from build123d import *

# Parameters (mm, degrees)
CROQUIS2_R              = 9.365
CROQUIS2_R_2            = 4.87
SALIENTE_EXTRUIR1_DEPTH = 0.2
CORTAR_EXTRUIR1_DEPTH   = 0.1


with BuildPart() as part:
    # Croquis2 → Saliente-Extruir1 (new body)
    with BuildSketch(Plane(origin=(0, 0, 0), x_dir=(1, 0, 0), z_dir=(0, 1, 0))):
        Circle(CROQUIS2_R)
        Circle(CROQUIS2_R_2, mode=Mode.SUBTRACT)
    extrude(amount=SALIENTE_EXTRUIR1_DEPTH)

    # Croquis3 → Cortar-Extruir1 (cut)
    with BuildSketch(Plane(origin=(0, 0.2, 0), x_dir=(1, 0, 0), z_dir=(0, 1, 0))):
        with BuildLine():
            Line((-0.5, 9.351642904), (-0.5, 4.84426465))
            ThreePointArc((-0.5, 4.84426465), (0, 4.87), (0.5, 4.84426465))
            Line((0.5, 4.84426465), (0.5, 9.351642904))
            ThreePointArc((0.5, 9.351642904), (0.25008919, 9.36166013), (0, 9.365))
            ThreePointArc((0, 9.365), (-0.25008919, 9.36166013), (-0.5, 9.351642904))
        make_face()
        with BuildLine():
            ThreePointArc((0.5, -4.84426465), (0, -4.87), (-0.5, -4.84426465))
            Line((-0.5, -4.84426465), (-0.5, -9.351642904))
            ThreePointArc((-0.5, -9.351642904), (-0.25008919, -9.36166013), (0, -9.365))
            ThreePointArc((0, -9.365), (0.25008919, -9.36166013), (0.5, -9.351642904))
            Line((0.5, -9.351642904), (0.5, -4.84426465))
        make_face()
        with BuildLine():
            Line((-4.84426465, 0.5), (-9.351642904, 0.5))
            ThreePointArc((-9.351642904, 0.5), (-9.36166013, 0.25008919), (-9.365, 0))
            ThreePointArc((-9.365, 0), (-9.36166013, -0.25008919), (-9.351642904, -0.5))
            Line((-9.351642904, -0.5), (-4.84426465, -0.5))
            ThreePointArc((-4.84426465, -0.5), (-4.87, 0), (-4.84426465, 0.5))
        make_face()
        with BuildLine():
            Line((9.351642904, 0.5), (4.84426465, 0.5))
            ThreePointArc((4.84426465, 0.5), (4.863561907, 0.250330935), (4.87, 0))
            ThreePointArc((4.87, 0), (4.863561907, -0.250330935), (4.84426465, -0.5))
            Line((4.84426465, -0.5), (9.351642904, -0.5))
            ThreePointArc((9.351642904, -0.5), (9.36166013, -0.25008919), (9.365, 0))
            ThreePointArc((9.365, 0), (9.36166013, 0.25008919), (9.351642904, 0.5))
        make_face()
        with BuildLine():
            ThreePointArc((6.622055006, 6.622055006), (6.442853599, 6.796533124), (6.259056722, 6.966163503))
            Line((6.259056722, 6.966163503), (4.854288053, 5.561394834))
            Line((4.854288053, 5.561394834), (5.561394834, 4.854288053))
            Line((5.561394834, 4.854288053), (6.966163503, 6.259056722))
            ThreePointArc((6.966163503, 6.259056722), (6.796533124, 6.442853599), (6.622055006, 6.622055006))
        make_face()
        with BuildLine():
            Line((4.854288053, -5.561394834), (6.259056722, -6.966163503))
            ThreePointArc((6.259056722, -6.966163503), (6.442853599, -6.796533124), (6.622055006, -6.622055006))
            ThreePointArc((6.622055006, -6.622055006), (6.796533124, -6.442853599), (6.966163503, -6.259056722))
            Line((6.966163503, -6.259056722), (5.561394834, -4.854288053))
            Line((5.561394834, -4.854288053), (4.854288053, -5.561394834))
        make_face()
        with BuildLine():
            Line((-5.561394834, -4.854288053), (-6.966163503, -6.259056722))
            ThreePointArc((-6.966163503, -6.259056722), (-6.796533124, -6.442853599), (-6.622055006, -6.622055006))
            ThreePointArc((-6.622055006, -6.622055006), (-6.442853599, -6.796533124), (-6.259056722, -6.966163503))
            Line((-6.259056722, -6.966163503), (-4.854288053, -5.561394834))
            Line((-4.854288053, -5.561394834), (-5.561394834, -4.854288053))
        make_face()
        Polygon((-4.854288053, 5.561394834), (-5.561394834, 4.854288053), (-6.975608396, 6.268501615), (-6.268501615, 6.975608396), align=None)
    extrude(amount=-CORTAR_EXTRUIR1_DEPTH, mode=Mode.SUBTRACT)


solid = part.part
Geometry: final body of the model. Coordinates: model frame, mm. Give positions to 0.01 mm unless a question says otherwise; leave off trailing zeros. Write each loop counter-clockwise with the first axis right and the second up, starting at its lowest first coordinate (ties: lowest second). Pieces come first, ordered by that corner, then holes. Notation, with made-up numbers: M 46.5,26.5 L 100.5,26.5 A20 ccw 100.5,33.5 Z; hole C 9.25,64.5 d7. An arc over 180 degrees is marked long. Answer in a Markdown table with one row per item. Add a question column.
(1) Section A-A on z = 0. Return loops of the section in (x, y) (3 decimals), and give its area (3 significant figures).
(2) Section C-C on y = 0.15. State how many separate pieces and enclosed holes the cut face has, and give its area (3 significant figures).
(3) Section B-B on x = 0. Return loops of the section in (y, z) (3 decimals), and give its area (3 significant figures).
(4) Ray query, line 1 (X direction, y = 0.15, z = 5.5); line 2 (Z direction, x = -0.25, y = 0.05); line 3 (Z direction, x = 7, y = 0.15). Return the intervals inside material, ascending.
(5) Section D-D on x = 7.5. Return loops of the section in (y, z), and give its area (3 significant figures).
(6) First-contact query: pin 1 (0.8 mm diameter, centred on x = 7, z = 0, fed in from +Y). Flat tip, straight axial feed; report the tip coordinate or a pass-through.
Result set:
| question | item | result |
|---|---|---|
| 1 | outline | M -9.365,0 L -4.87,0 L -4.87,0.1 L -9.365,0.1 Z; M 4.87,0 L 9.365,0 L 9.365,0.1 L 4.87,0.1 Z |
| 1 | area | 0.899 mm^2 |
| 2 | separate pieces | 4 |
| 2 | enclosed holes | 0 |
| 2 | area | 175 mm^2 |
| 3 | outline | M 0,-9.365 L 0.1,-9.365 L 0.1,-4.87 L 0,-4.87 Z; M 0,4.87 L 0.1,4.87 L 0.1,9.365 L 0,9.365 Z |
| 3 | area | 0.899 mm^2 |
| 4 | line 1 | x = -7.58 to -6.21, -4.92 to -0.5, 0.5 to 4.92, 6.21 to 7.58 |
| 4 | line 2 | z = -9.36 to -4.86, 4.86 to 9.36 |
| 4 | line 3 | z = -6.22 to -0.5, 0.5 to 6.22 |
| 5 | outline | M 0,-5.61 L 0.2,-5.61 L 0.2,-0.5 L 0.1,-0.5 L 0.1,0.5 L 0.2,0.5 L 0.2,5.61 L 0,5.61 Z |
| 5 | area | 2.14 mm^2 |
| 6 | pin 1 | stops at y = 0.1 |
